from build123d import *

# Parameters (mm, degrees)
SKETCH_1_R      = 2
SKETCH_1_R_2    = 0.5
EXTRUDE_2_DEPTH = 1
SKETCH_2_R      = 3.5
SKETCH_2_R_2    = 2
EXTRUDE_3_DEPTH = 3


with BuildPart() as part:
    # 草图1 → 凸台-拉伸2 (new body)
    with BuildSketch(Plane.XY):
        with BuildLine():
            Line((14.650323726, 1.492448585), (2.165063509, 2.75))
            ThreePointArc((2.165063509, 2.75), (-3.5, 0), (2.165063509, -2.75))
            Line((2.165063509, -2.75), (14.650323726, -1.492448585))
            ThreePointArc((14.650323726, -1.492448585), (16, 0), (14.650323726, 1.492448585))
        make_face()
        Circle(SKETCH_1_R, mode=Mode.SUBTRACT)
        with Locations((14.5, 0)):
            Circle(SKETCH_1_R_2, mode=Mode.SUBTRACT)
    extrude_2 = extrude(amount=EXTRUDE_2_DEPTH)

    # 草图2 → 凸台-拉伸3 (add)
    with BuildSketch(Plane.XY.offset(1)):
        Circle(SKETCH_2_R)
        Circle(SKETCH_2_R_2, mode=Mode.SUBTRACT)
    extrude(amount=EXTRUDE_3_DEPTH)

    # 镜向1: 凸台-拉伸2 across plane
    add(extrude_2.mirror(Plane(origin=(0, 0, 0), x_dir=(0, 0, 1), z_dir=(1, 0, 0))))


solid = part.part
The listing builds one solid part. Answer for the finished solid, in the listing's coordinates (mm). Round coordinates to 2 decimals unless told otherwise and drop trailing zeros. Loops run counter-clockwise (first coordinate to the right, second up) from the corner with the lowest first, then second, coordinate; pieces in that order, holes last. Notation, with made-up numbers: M 45.5,87 L 50.5,87 A12 cw 50.5,98 Z; hole C 39,-37.75 d11. An arc over 180 degrees is marked long. Return JSON: item names as keys, results as strings.
Q1. Each of these flat-tipped pins is pushed along its axis until it touches: pin 1 Ø4 at (x, y) = (12, 1.5) entering from +Z; pin 2 Ø2 at (y, z) = (2, 3) entering from +X; pin 3 Ø1.5 at (y, z) = (-2, 2) entering from +X. Where does it stop, or does it pass through?
Results list:
{"pin 1": "stops at z = 1", "pin 2": "stops at x = 3.35", "pin 3": "stops at x = 3.27"}
Q2. The mould has two halves that part along Y. Classify faces 1 (the face through (-14.962, -0.192, 0.493)), 2 (the face through (-8.5, 2.11, 0.49)), 3 (the face through (2, -2, 4)), 4 (the face through (16, 0, 0.5)): released by +Y, released by -Y, zero draft, split by the parting line, or undercut.
Results list:
{"face 1": "undercut", "face 2": "released by +Y", "face 3": "zero draft", "face 4": "split by the parting line"}
Q3. Find section C-C, the plane z = 3.3. Determine the outline of the cut face in (x, y), plus the area to 3 significant figures.
Results list:
{"outline": "C 0,0 d7; hole C 0,0 d4", "area": "25.9 mm2"}
Q4. Find section D-D, the plane x = 12. Determine the outline of the cut face in (y, z), plus the area to 3 significant figures.
Results list:
{"outline": "M -1.76,0 L 1.76,0 L 1.76,1 L -1.76,1 Z", "area": "3.52 mm2"}
Q5. Find section B-B, the plane x = 0. Determine the outline of the cut face in (y, z), plus the area to 3 significant figures.
Results list:
{"outline": "M -3.5,0 L -2,0 L -2,4 L -3.5,4 Z; M 2,0 L 3.5,0 L 3.5,4 L 2,4 Z", "area": "12.0 mm2"}
Q6. Find the intervals of material crossed by line 1 along Y through (x, z) = (0, 2.1); line 2 along Z through (x, y) = (6.5, 0.5); line 3 along Y through (x, z) = (-14.5, 0.8), in increasing order. Write a range as from..to.
Results list:
{"line 1": "y = -3.5..-2, 2..3.5", "line 2": "z = 0..1", "line 3": "y = -1.51..-0.5, 0.5..1.51"}
Q7. Find section A-A, the plane y = 0. Determine the outline of the cut face in (x, z).
Results list:
{"outline": "M -16,0 L -15,0 L -15,1 L -16,1 Z; M -14,0 L -2,0 L -2,4 L -3.5,4 L -3.5,1 L -14,1 Z; M 2,0 L 14,0 L 14,1 L 3.5,1 L 3.5,4 L 2,4 Z; M 15,0 L 16,0 L 16,1 L 15,1 Z"}
